Autodesk Inventor part; units mm, degrees
ref_plane "YZ Plane" through (0, 0, 0) normal (1, 0, 0) x (0, 1, 0)
ref_plane "XZ Plane" through (0, 0, 0) normal (0, 1, 0) x (-1, 0, 0)
ref_plane "XY Plane" through (0, 0, 0) normal (0, 0, 1) x (1, 0, 0)
sketch "Sketch1" plane through (0, 0, 0) normal (1, 0, 0) x (0, 1, 0)
  line L0 (0, 0) -> (0, -17.78)
  line L1 (0, -17.78) -> (7.62, -17.78)
  line L2 (7.62, -17.78) -> (7.62, -14.986)
  line L3 (0, 0) -> (7.62, 0)
  line L4 (7.62, 0) -> (7.62, -2.794)
  line L5 (3.81, -13.589) -> (3.81, -4.191)
  arc A0 (7.112, -4.191) -> (4.3826, -3.7711) centre (5.715, -4.191) ccw
  arc A1 (4.3826, -14.0089) -> (7.112, -13.589) centre (5.715, -13.589) ccw
  line L6 (7.62, -2.794) -> (7.62, -4.191)
  line L7 (7.62, -4.191) -> (7.112, -4.191)
  line L8 (7.62, -14.986) -> (7.62, -13.589)
  line L9 (7.62, -13.589) -> (7.112, -13.589)
  line L10 (3.81, -4.191) -> (4.3826, -3.7711)
  line L11 (3.81, -13.589) -> (4.3826, -14.0089)
  dimension "d3" = 17.78
  dimension "d4" = 7.62
  dimension "d6" = 2.794
extrude "Extrusion1" add sketch "Sketch1" along normal blind 5.08
equation "\"d6\" = d5"
properties part number "led_clip"
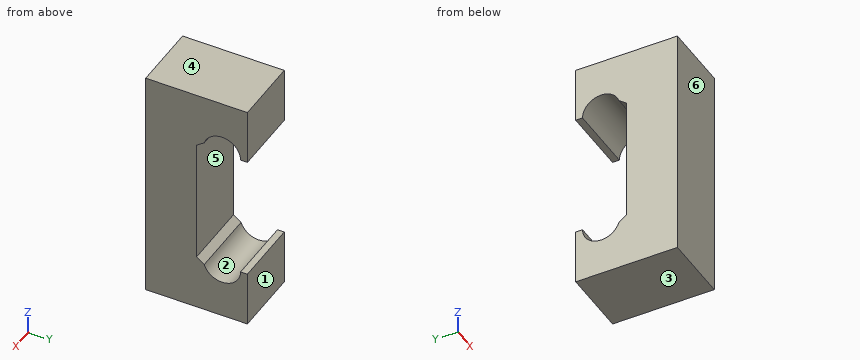
Could you check a few things on this model? Use its own coordinates, in mm. Face numbers are marked on the shaded views. A direction names the side the tool comes from. Coordinates: 2 decimals unless noted, no trailing zeros. Order: outer loops, then holes, each group sorted by start corner. A loop starts at its lowest first (then second) coordinate and runs counter-clockwise, first axis right, second up. Notation, with made-up numbers: (1, 32.5) -> (51, 32.5) arc R22 cw to (51, 41.5) -> close; hole circle Ø7 at (76, 27.5). An arc over 180 degrees is marked (long way). One line per item, written item: value. Start each with the question number.
1) Imagine slicing it at B-B on z = -13.75. List the corners of the cut face in (x, y) for me, plus the area to 3 significant figures.
2) We'd pull the mould along Z, two halves only. Please class the marked faces 3, 4, 5 and 6: +Z half, -Z half, draft (parallel to the pull), parting line (faces both ways), or undercut.
3) Which directions (+Z, -Z, +X, -X, +Y, -Y) give clear straight access to the entire face, cutting with the end or side of a thin tool? Please do the marked faces 1 and 2.
4) If I drill on L1, parallel to Z at x = 1.9, y = 7.25; L2, parallel to Z at x = 1.4, y = 5.75; L3, parallel to Y at x = 4.85, z = -14.5, over which ranges is the centre line in solid material (lowest first)? Write a range as [from, to].
5) Imagine slicing it at C-C on x = 2.95. List the corners of the cut face in (y, z) for me (3 decimals).
6) I'm going to push a flat-ended pin straight in: pin 1 (1 mm diameter, centred on y = 5.5, z = -14, fed in from -X). Where does the tip first touch, or does it pass through?
7) Imagine slicing it at D-D on z = -10.75. List the corners of the cut face in (x, y) for me, plus the area to 3 significant figures.
8) Imagine slicing it at A-A on y = 6.25. List the corners of the cut face in (x, z) for me.
Answer list:
1. outline: (0, 0) -> (5.08, 0) -> (5.08, 4.03) -> (0, 4.03) -> close; (0, 7.1) -> (5.08, 7.1) -> (5.08, 7.62) -> (0, 7.62) -> close
1. area: 23.1 mm2
2. face 3: -Z half
2. face 4: +Z half
2. face 5: undercut
2. face 6: draft
3. face 1: +Z, -Z, +X, -X, +Y
3. face 2: +X, -X
4. L1: z = [-17.78, -13.59], [-4.19, 0]
4. L2: z = [-17.78, -14.99], [-2.79, 0]
4. L3: y = [0, 4.66], [6.77, 7.62]
5. outline: (0, -17.78) -> (7.62, -17.78) -> (7.62, -13.589) -> (7.112, -13.589) arc R1.397 cw to (4.383, -14.009) -> (3.81, -13.589) -> (3.81, -4.191) -> (4.383, -3.771) arc R1.397 cw to (7.112, -4.191) -> (7.62, -4.191) -> (7.62, 0) -> (0, 0) -> close
6. pin 1: passes through
7. outline: (0, 0) -> (5.08, 0) -> (5.08, 3.81) -> (0, 3.81) -> close
7. area: 19.4 mm2
8. outline: (0, -17.78) -> (5.08, -17.78) -> (5.08, -14.88) -> (0, -14.88) -> close; (0, -2.9) -> (5.08, -2.9) -> (5.08, 0) -> (0, 0) -> close
